from build123d import *

# Parameters (mm, degrees)
SKETCH1_R           = 4
BOSS_EXTRUDE1_DEPTH = 329.2
SKETCH2_R           = 6
BOSS_EXTRUDE2_DEPTH = 282
SKETCH4_R           = 5
SKETCH4_R_2         = 4
CUT_EXTRUDE1_DEPTH  = 30


with BuildPart() as part:
    # Sketch1 → Boss-Extrude1 (new body)
    with BuildSketch(Plane(origin=(0, 0, 0), x_dir=(1, 0, 0), z_dir=(0, 1, 0))):
        Circle(SKETCH1_R)
    extrude(amount=BOSS_EXTRUDE1_DEPTH)

    # Sketch2 → Boss-Extrude2 (add)
    with BuildSketch(Plane(origin=(0, 326.2, 0), x_dir=(1, 0, 0), z_dir=(0, 1, 0))):
        Circle(SKETCH2_R)
    extrude(amount=-BOSS_EXTRUDE2_DEPTH)

    # Sketch4 → Cut-Extrude1 (cut)
    with BuildSketch(Plane(origin=(0, 289.2, 0), x_dir=(1, 0, 0), z_dir=(0, 1, 0))):
        Circle(SKETCH4_R)
        Circle(SKETCH4_R_2, mode=Mode.SUBTRACT)
    extrude(amount=-CUT_EXTRUDE1_DEPTH, mode=Mode.SUBTRACT)


solid = part.part
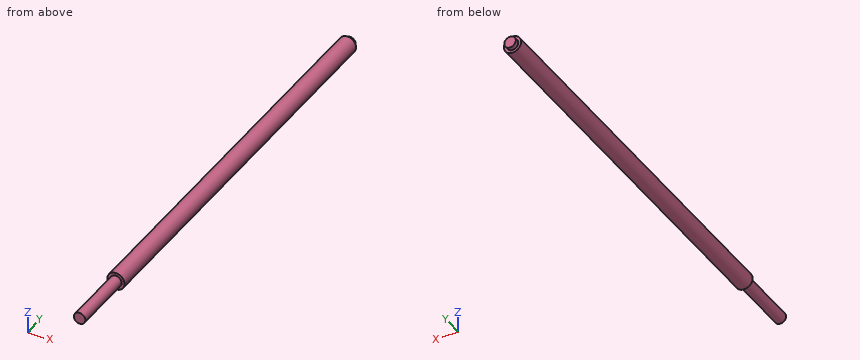
Could you check a few things on this model? Use its own coordinates, in mm. Give positions to 0.01 mm unless a question says otherwise; leave off trailing zeros. Loops run counter-clockwise (first coordinate to the right, second up) from the corner with the lowest first, then second, coordinate; pieces in that order, holes last. Notation, with made-up numbers: (-38.5, 83) -> (-25.5, 83) arc R31 ccw to (-25.5, 118) -> close; hole circle Ø5 at (48, -22.5). An arc over 180 degrees is marked (long way). Return JSON: item names as keys, results as strings.
Item 1: I need wall thicknesses on L1, parallel to Z at x = 0, y = 278.75; L2, parallel to Y at x = 3.25, z = -3. Which ranges of each line are inside material? Lowest first, please. Write a range as from..to.
Geometry results:
{"L1": "z = -6..-5, -4..4, 5..6", "L2": "y = 44.2..259.2, 289.2..326.2"}
Item 2: I'm going to push flat-ended pins straight in: pin 1 (2 mm diameter, centred on x = -1.5, y = 187.5, fed in from -Z); pin 2 (5 mm diameter, centred on y = 167, z = 3.5, fed in from +X); pin 3 (2 mm diameter, centred on x = -3.5, y = 224.5, fed in from -Z). Where does each tip first touch, or does it pass through?
Geometry results:
{"pin 1": "stops at z = -5.98", "pin 2": "stops at x = 5.92", "pin 3": "stops at z = -5.45"}
Item 3: If we section it at A-A on z = 0: List the corners of the cut face in (x, y) for me, plus the area to 3 significant figures.
Geometry results:
{"outline": "(-6, 44.2) -> (-4, 44.2) -> (-4, 0) -> (4, 0) -> (4, 44.2) -> (6, 44.2) -> (6, 326.2) -> (4, 326.2) -> (4, 329.2) -> (-4, 329.2) -> (-4, 326.2) -> (-6, 326.2) -> close; hole (-5, 259.2) -> (-4, 259.2) -> (-4, 289.2) -> (-5, 289.2) -> close; hole (4, 259.2) -> (5, 259.2) -> (5, 289.2) -> (4, 289.2) -> close", "area": "3,700 mm²"}
Item 4: If we section it at B-B on x = 0: List the corners of the cut face in (y, z) for me.
Geometry results:
{"outline": "(0, -4) -> (44.2, -4) -> (44.2, -6) -> (326.2, -6) -> (326.2, -4) -> (329.2, -4) -> (329.2, 4) -> (326.2, 4) -> (326.2, 6) -> (44.2, 6) -> (44.2, 4) -> (0, 4) -> close; hole (259.2, -5) -> (289.2, -5) -> (289.2, -4) -> (259.2, -4) -> close; hole (259.2, 4) -> (289.2, 4) -> (289.2, 5) -> (259.2, 5) -> close"}
Item 5: If we section it at C-C on y = 147.5: List the corners of the cut face in (x, z) for me, plus the area to 3 significant figures.
Geometry results:
{"outline": "circle Ø12 at (0, 0)", "area": "113 mm²"}
